```python
from build123d import *

# Parameters (mm, degrees)
F0_W        = 88.9418646693
F0_H        = 98.6094549298
F1_DEPTH    = 12.7
F2_W        = 80.0476707518
F2_H        = 5.413854029
F3_DEPTH    = 76.2
F4_T1_DEPTH = 124.7377540876
F4_T3_DEPTH = 115.0701638271


# Not quite as in the source:
# - a fillet or chamfer that OpenCascade refuses, or shapes differently, is made with other operations: its cross-section is extruded or revolved along the edge and cut away or added


with BuildPart() as f1:
    # F0 (on Front) → F1 (new body)
    with BuildSketch(Plane.XZ):
        Rectangle(F0_W, F0_H)
    extrude(amount=F1_DEPTH)

    # F2 (on face) → F3 (cut)
    with BuildSketch(Plane.XY.offset(49.3047274649)):
        with Locations((-1.8626e-06, -6.1872594524)):
            Rectangle(F2_W, F2_H)
    extrude(amount=-F3_DEPTH, mode=Mode.SUBTRACT)

    # F4: chamfer of 5.08 on 8 edges, made by hand

    # F4_s2 → F4_t1 (cut)
    with BuildSketch(Plane.XY.offset(-62.3688770438)):
        Polygon((44.4709323347, -5.08), (39.3909323347, 0), (44.4709323347, 0), align=None)
        Polygon((-39.3909323347, 0), (-44.4709323347, -5.08), (-44.4709323347, 0), align=None)
        Polygon((44.4709323347, -7.62), (39.3909323347, -12.7), (44.4709323347, -12.7), align=None)
        Polygon((-39.3909323347, -12.7), (-44.4709323347, -7.62), (-44.4709323347, -12.7), align=None)
    extrude(amount=F4_T1_DEPTH, mode=Mode.SUBTRACT)

    # F4_s4 → F4_t3 (cut)
    with BuildSketch(Plane.YZ.offset(-57.5350819135)):
        Polygon((-5.08, 49.3047274649), (0, 44.2247274649), (0, 49.3047274649), align=None)
        Polygon((-5.08, -49.3047274649), (0, -44.2247274649), (0, -49.3047274649), align=None)
        Polygon((-7.62, 49.3047274649), (-12.7, 44.2247274649), (-12.7, 49.3047274649), align=None)
        Polygon((-7.62, -49.3047274649), (-12.7, -44.2247274649), (-12.7, -49.3047274649), align=None)
    extrude(amount=F4_T3_DEPTH, mode=Mode.SUBTRACT)


solid = f1.part
```
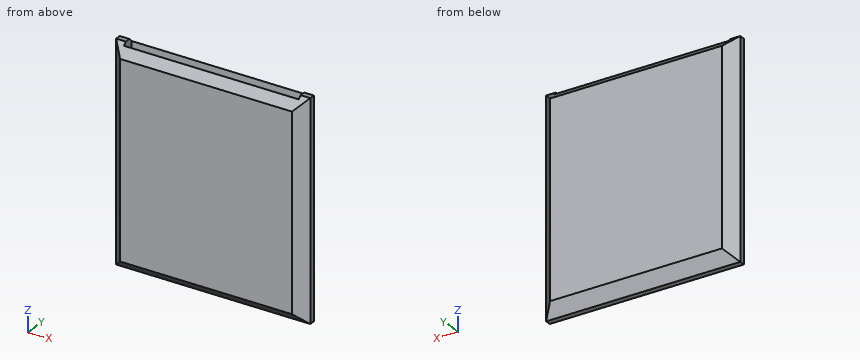
Verification items for the finished model (mm, model axes). Coordinates: 2 decimals unless noted, no trailing zeros. Loops run counter-clockwise (first coordinate to the right, second up) from the corner with the lowest first, then second, coordinate; pieces in that order, holes last. Notation, with made-up numbers: (-35.5, 59.5) -> (-21.5, 59.5) arc R16 cw to (-21.5, 86.5) -> close; hole circle Ø7 at (52.25, 35). An arc over 180 degrees is marked (long way). Answer in a Markdown table with one row per item. Add a question column.
1. Depth check by flat-ended pin: P1, Ø1.5, axis at x = -0.5, y = -10.5, coming from the -Z side; P2, Ø2.5, axis at x = 3.5, y = -7, coming from the +Z side; P3, Ø1.5, axis at y = -3.5, z = -21, coming from the +X side. Enter the tip coordinate at first touch or a pass-through.
2. Section check B-B, the plane x = 24. Enter the section's corners in (y, z), then the cut area to 3 significant figures.
3. Material ranges on probe 1 along Y at (x, z) = (-10.5, 18.5); probe 2 along X at (y, z) = (-6, 37); probe 3 along X at (y, z) = (-8, 32), recorded low to high. Write a range as [from, to].
4. Section check C-C, the plane z = -33. Enter the section's corners in (x, y), then the cut area to 3 significant figures.
5. Section check A-A, the plane z = 36.5. Enter the section's corners in (x, y), then the cut area to 3 significant figures.
6. Section check D-D, the plane y = -2. Enter the section's corners in (x, z).
Derived:
| question | item | result |
|---|---|---|
| 1 | P1 | stops at z = -47.17 |
| 1 | P2 | stops at z = -26.9 |
| 1 | P3 | stops at x = 43.64 |
| 2 | outline | (-12.7, -44.22) -> (-7.62, -49.3) -> (-5.08, -49.3) -> (0, -44.22) -> (0, 44.22) -> (-3.48, 47.71) -> (-3.48, -26.9) -> (-8.89, -26.9) -> (-8.89, 48.03) -> (-12.7, 44.22) -> close |
| 2 | area | 790 mm² |
| 3 | probe 1 | y = [-12.7, -8.89], [-3.48, 0] |
| 3 | probe 2 | x = [-44.47, -40.02], [40.02, 44.47] |
| 3 | probe 3 | x = [-44.09, -40.02], [40.02, 44.09] |
| 4 | outline | (-44.47, -7.62) -> (-39.39, -12.7) -> (39.39, -12.7) -> (44.47, -7.62) -> (44.47, -5.08) -> (39.39, 0) -> (-39.39, 0) -> (-44.47, -5.08) -> close |
| 4 | area | 1,080 mm² |
| 5 | outline | (-44.47, -7.62) -> (-39.39, -12.7) -> (39.39, -12.7) -> (44.47, -7.62) -> (44.47, -5.08) -> (39.39, 0) -> (-39.39, 0) -> (-44.47, -5.08) -> close; hole (-40.02, -8.89) -> (40.02, -8.89) -> (40.02, -3.48) -> (-40.02, -3.48) -> close |
| 5 | area | 645 mm² |
| 6 | outline | (-41.39, -46.22) -> (41.39, -46.22) -> (41.39, 46.22) -> (-41.39, 46.22) -> close |
